Geometry: final body of the model. Coordinates: model frame, mm. Face numbers are marked on the shaded views. Coordinates: 2 decimals unless noted, no trailing zeros. Write each loop counter-clockwise with the first axis right and the second up, starting at its lowest first coordinate (ties: lowest second). Pieces come first, ordered by that corner, then holes. Notation, with made-up numbers: (74.25, 81) -> (119.25, 81) arc R22 cw to (119.25, 97) -> close; hole circle Ø11 at (11.5, 17.5). An arc over 180 degrees is marked (long way). One line per item, written item: value. Start each with the question number.
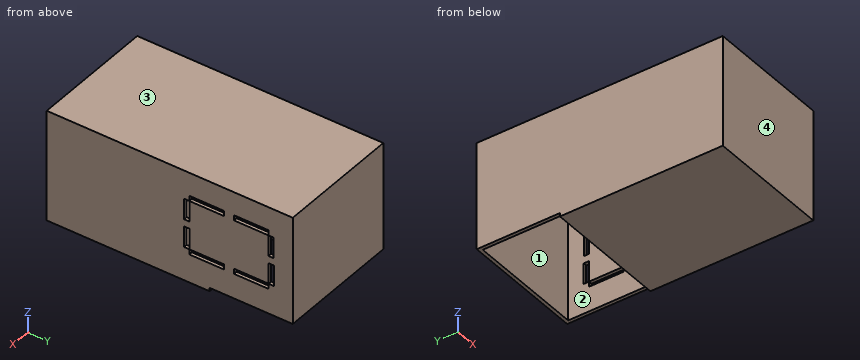
Autodesk Inventor part; units mm, degrees
ref_plane "YZ Plane" through (0, 0, 0) normal (1, 0, 0) x (0, 1, 0)
ref_plane "XZ Plane" through (0, 0, 0) normal (0, 1, 0) x (-1, 0, 0)
ref_plane "XY Plane" through (0, 0, 0) normal (0, 0, 1) x (1, 0, 0)
sketch "Sketch1" plane through (0, 0, 0) normal (1, 0, 0) x (0, 1, 0)
  line L0 (11.3212, 0) -> (-338.6788, 0)
  line L1 (-338.6788, 0) -> (-338.6788, 150)
  line L2 (-338.6788, 150) -> (11.3212, 150)
  line L3 (11.3212, 150) -> (11.3212, 0)
  point P0 (0, 0)
  dimension "d0" = 350
  dimension "d1" = 150
extrude "Extrusion1" add sketch "Sketch1" along normal blind 5
sketch "Sketch2" plane through (5, 0, 0) normal (1, 0, 0) x (0, 0, -1)
  line L0 (-150, 11.3212) -> (-150, -338.6788)
  line L1 (0, -338.6788) -> (0, 11.3212)
  line L2 (-150, 11.3212) -> (0, 11.3212)
  line L3 (0, 11.3212) -> (0, 6.3212)
  line L4 (0, 6.3212) -> (-150, 6.3212)
  line L5 (-150, 6.3212) -> (-150, 11.3212)
  point P0 (0, 0)
  point P1 (0, 11.3212)
  dimension "d4" = 5
extrude "Extrusion2" add sketch "Sketch2" along normal blind 170
sketch "Sketch3" plane through (0, -338.6788, 150) normal (0, 0, 1) x (1, 0, 0)
  point P0 (0, 338.6788)
sketch "Sketch4" plane through (0, -338.6788, 150) normal (0, 0, 1) x (1, 0, 0)
  line L0 (0, 350) -> (0, 0)
  line L1 (0, 350) -> (175.2508, 350)
  line L2 (175.2508, 350) -> (175.2508, 0)
  line L3 (175.2508, 0) -> (0, 0)
  line L4 (0, 0) -> (0, 350)
  point P0 (0, 338.6788)
extrude "Extrusion3" add sketch "Sketch4" along normal blind 5
sketch "Sketch5" plane through (175, 0, 0) normal (1, 0, 0) x (0, 0, -1)
  line L0 (0, 11.3212) -> (-155, 11.3212)
  line L1 (-155, 11.3212) -> (0, 11.3212)
  line L2 (0, 11.3212) -> (0, -338.6788)
  line L3 (0, -338.6788) -> (-155, -338.6788)
  line L4 (-155, -338.6788) -> (-155, 11.3212)
  point P0 (0, 0)
extrude "Extrusion4" add sketch "Sketch5" along normal blind 5
sketch "Sketch6" plane through (0, -338.6788, 0) normal (0, 0, -1) x (-1, 0, 0)
  line L0 (-180, 0) -> (-180, 350)
  line L1 (-180, 0) -> (0, 0)
  line L2 (0, 0) -> (0, 230)
  line L3 (0, 230) -> (-180, 230)
  line L4 (-180, 230) -> (-180, 0)
  point P0 (0, 338.6788)
  point P1 (-180, 230)
  dimension "d34" = 230
extrude "Extrusion5" add sketch "Sketch6" along normal blind 5
sketch "Sketch7" plane through (0, -338.6788, 155) normal (0, -1, 0) x (1, 0, 0)
  line L0 (180, -155) -> (180, 0)
  line L1 (0, -160) -> (180, -160)
  line L2 (180, 0) -> (0, 0)
  line L3 (0, 0) -> (0, -160)
  line L4 (0, -160) -> (180, -160)
  line L5 (180, -160) -> (180, 0)
  point P0 (0, -155)
extrude "Extrusion6" add sketch "Sketch7" along normal blind 5
sketch "Sketch8" plane through (180, 0, 0) normal (1, 0, 0) x (0, 0, -1)
  point P0 (0, 0)
sketch "Sketch9" plane through (180, 0, 0) normal (1, 0, 0) x (0, 0, -1)
  line L0 (-113.8942, -23.5999) -> (-43.3942, -23.5999)
  line L1 (-43.3942, -23.5999) -> (-43.3942, -137.9783)
  line L2 (-43.3942, -137.9783) -> (-113.8942, -137.9783)
  line L3 (-113.8942, -137.9783) -> (-113.8942, -23.5999)
  line L4 (-43.3942, -73.5999) -> (-43.3942, -23.5999)
  line L5 (-43.3942, -137.9783) -> (-35.8942, -137.9783)
  line L6 (-35.8942, -137.9783) -> (-35.8942, -87.9783)
  line L7 (-35.8942, -87.9783) -> (-43.3942, -87.9783)
  line L8 (-43.3942, -87.9783) -> (-43.3942, -137.9783)
  line L9 (-43.3942, -65.8129) -> (-43.3942, -23.5999)
  line L10 (-113.8942, -23.5999) -> (-121.3942, -23.5999)
  line L11 (-121.3942, -23.5999) -> (-121.3942, -73.5999)
  line L12 (-121.3942, -73.5999) -> (-113.8942, -73.5999)
  line L13 (-113.8942, -73.5999) -> (-113.8942, -23.5999)
  line L14 (-113.8942, -137.9783) -> (-121.3942, -137.9783)
  line L15 (-121.3942, -137.9783) -> (-121.3942, -87.9783)
  line L16 (-121.3942, -87.9783) -> (-113.8942, -87.9783)
  line L17 (-113.8942, -87.9783) -> (-113.8942, -137.9783)
  line L18 (-113.8942, -137.9783) -> (-83.8942, -137.9783)
  line L19 (-83.8942, -137.9783) -> (-83.8942, -145.4783)
  line L20 (-83.8942, -145.4783) -> (-113.8942, -145.4783)
  line L21 (-113.8942, -145.4783) -> (-113.8942, -137.9783)
  line L22 (-43.3942, -137.9783) -> (-73.3942, -137.9783)
  line L23 (-73.3942, -137.9783) -> (-73.3942, -145.4783)
  line L24 (-73.3942, -145.4783) -> (-43.3942, -145.4783)
  line L25 (-43.3942, -145.4783) -> (-43.3942, -137.9783)
  line L26 (-43.3942, -23.5999) -> (-35.8942, -23.5999)
  line L27 (-35.8942, -23.5999) -> (-35.8942, -73.5999)
  line L28 (-35.8942, -73.5999) -> (-43.3942, -73.5999)
  line L29 (-43.3942, -73.5999) -> (-43.3942, -23.5999)
  line L30 (-113.8942, -23.5999) -> (-83.8942, -23.5999)
  line L31 (-83.8942, -23.5999) -> (-83.8942, -16.6897)
  line L32 (-83.8942, -16.6897) -> (-113.8942, -16.6897)
  line L33 (-113.8942, -16.6897) -> (-113.8942, -23.5999)
  line L34 (-73.3942, -16.0999) -> (-43.3942, -16.0999)
  line L35 (-43.3942, -16.0999) -> (-43.3942, -23.5999)
  line L36 (-43.3942, -23.5999) -> (-73.3942, -23.5999)
  line L37 (-73.3942, -23.5999) -> (-73.3942, -16.0999)
  point P0 (0, 0)
  dimension "d18" = 7.5
  dimension "d19" = 7.5
  dimension "d20" = 30
  dimension "d21" = 30
  dimension "d22" = 7.5
  dimension "d23" = 50
  dimension "d24" = 50
  dimension "d25" = 50
  dimension "d26" = 50
  dimension "d27" = 7.5
  dimension "d28" = 7.5
  dimension "d29" = 30
  dimension "d30" = 30
  dimension "d31" = 7.5
extrude "Extrusion7" cut sketch "Sketch9" against normal blind 5 contours L33 L32 L31 L0 | L3 L12 L11 L10 | L37 L34 L35 L0 | L3 L14 L15 L16 | L26 L27 L28 L1 | L2 L19 L20 L21 | L2 L25 L24 L23 | L7 L6 L5 L1
sketch "Sketch10" plane through (180, 0, 0) normal (1, 0, 0) x (0, 0, -1)
  point P0 (0, 0)
properties part number "button unit" material "Pine, Southern"
Q1. Cut plane A-A on y = -244.5. Output: boundary loops of the cut face in (x, z).
Q2. Cut plane B-B on z = 89. Output: boundary loops of the cut face in (x, y), and give its area (3 significant figures).
Q3. Cut plane D-D on z = 15. Output: boundary loops of the cut face in (x, y), and give its area (3 significant figures).
Q4. First-contact query: P1, Ø1.5, axis at x = 74, z = -2, coming from the +Y side; P2, Ø5.5, axis at x = 178.5, y = -52, coming from the -Z side. Flat tips, straight axial feed; report the tip coordinate or a pass-through.
Q5. Cut plane C-C on x = 54. Output: boundary loops of the cut face in (y, z), and give its area (3 significant figures).
Q6. Line query: L1, parallel to X at y = -31.5, z = 97; L2, parallel to Z at x = 98, y = -123.5; L3, parallel to Y at x = 85, z = 16.5. Output: solid intervals per line, ascending. Write a range as from..to.
Q7. Draft query along Y for the marked faces 1, 2, 3 and 4. Return one class per face: pulls with the +Y half, pulls with the -Y half, needs draft (parallel to the pull), parting line crosses it, or undercut.
Solution:
1. outline: (0, -5) -> (180, -5) -> (180, 155) -> (0, 155) -> close; hole (5, 0) -> (175, 0) -> (175, 150) -> (5, 150) -> close
2. outline: (0, -343.68) -> (180, -343.68) -> (180, -145.48) -> (175, -145.48) -> (175, -338.68) -> (5, -338.68) -> (5, 6.32) -> (175, 6.32) -> (175, -16.69) -> (180, -16.69) -> (180, 11.32) -> (0, 11.32) -> close; (175, -137.98) -> (180, -137.98) -> (180, -23.6) -> (175, -23.6) -> close
2. area: 5,180 mm²
3. outline: (0, -343.68) -> (180, -343.68) -> (180, 11.32) -> (0, 11.32) -> close; hole (5, -338.68) -> (175, -338.68) -> (175, 6.32) -> (5, 6.32) -> close
3. area: 5,250 mm²
4. P1: y = -108.68
4. P2: z = 0
5. outline: (-343.68, -5) -> (-108.68, -5) -> (-108.68, 0) -> (-338.68, 0) -> (-338.68, 150) -> (6.32, 150) -> (6.32, 0) -> (11.32, 0) -> (11.32, 155) -> (-343.68, 155) -> close
5. area: 4,450 mm²
6. L1: 0..5, 175..180
6. L2: -5..0, 150..155
6. L3: -343.68..-338.68, 6.32..11.32
7. face 1: undercut
7. face 2: undercut
7. face 3: needs draft
7. face 4: pulls with the -Y half
